Source: three-view drawing plus pictorial views. Frame: mm from the lowest corner of the part. A direction names the side the tool comes from. Give positions to 0.01 mm unless a question says otherwise; leave off trailing zeros. Write each loop counter-clockwise with the first axis right and the second up, starting at its lowest first coordinate (ties: lowest second). Pieces come first, ordered by that corner, then holes. Notation, with made-up numbers: (-20.5, 12.25) -> (24.5, 12.25) arc R22 cw to (24.5, 23.25) -> close; hole circle Ø6 at (2, -32.75). An arc over 180 degrees is marked (long way). Write item = value, one per line.
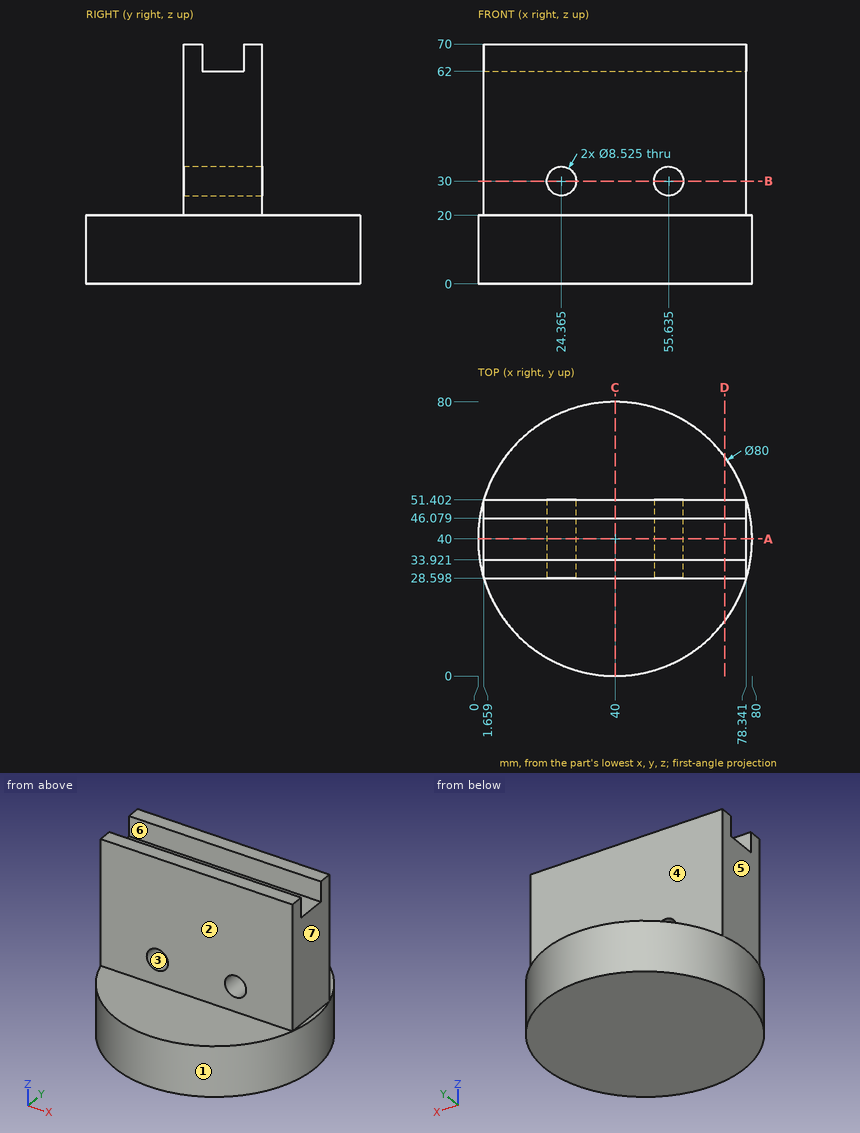
1) Contact query for flat-ended pins moving along their axis: pin 1 (5 mm diameter, centred on x = 11.5, z = 25, fed in from +Y); pin 2 (0.5 mm diameter, centred on x = 1, y = 38.5, fed in from +Z); pin 3 (11.5 mm diameter, centred on y = 36, z = 56, fed in from -X). Output: stop coordinate, or through.
Computed:
pin_1 = 51.4
pin_2 = 20
pin_3 = 1.66
2) Access query for the marked faces 4, 5, 6 and 7. Directions: +Z, -Z, +X, -X, +Y, -Y. A direction counts if a zero-diameter tool reaches every point of the face in a straight line with its end or side. Return the directions, or none.
Computed:
face_4 = +Z, +X, -X, +Y
face_5 = +Z, -X, +Y, -Y
face_6 = +Z, +X, -X
face_7 = +Z, +X, +Y, -Y
3) Cut plane A-A (y = 40). Return the cut outline in (x, z) (1 decimal), then the cut area to 3 significant figures.
Computed:
outline = (0, 0) -> (80, 0) -> (80, 20) -> (78.3, 20) -> (78.3, 62) -> (1.7, 62) -> (1.7, 20) -> (0, 20) -> close; hole circle Ø8.5 at (24.4, 30); hole circle Ø8.5 at (55.6, 30)
area = 4,710 mm²
4) Cut plane D-D (x = 72). Return the cut outline in (y, z).
Computed:
outline = (16, 0) -> (64, 0) -> (64, 20) -> (51.4, 20) -> (51.4, 70) -> (46.08, 70) -> (46.08, 62) -> (33.92, 62) -> (33.92, 70) -> (28.6, 70) -> (28.6, 20) -> (16, 20) -> close
5) Cut plane C-C (x = 40). Return the cut outline in (y, z), then the cut area to 3 significant figures.
Computed:
outline = (0, 0) -> (80, 0) -> (80, 20) -> (51.4, 20) -> (51.4, 70) -> (46.08, 70) -> (46.08, 62) -> (33.92, 62) -> (33.92, 70) -> (28.6, 70) -> (28.6, 20) -> (0, 20) -> close
area = 2,640 mm²
6) Cut plane B-B (z = 30). Return the cut outline in (x, y), then the cut area to 3 significant figures.
Computed:
outline = (1.66, 28.6) -> (20.1, 28.6) -> (20.1, 51.4) -> (1.66, 51.4) -> close; (28.63, 28.6) -> (51.37, 28.6) -> (51.37, 51.4) -> (28.63, 51.4) -> close; (59.9, 28.6) -> (78.34, 28.6) -> (78.34, 51.4) -> (59.9, 51.4) -> close
area = 1,360 mm²
7) Draft query along X for the marked faces 1, 2 and 3. Return one class per face: pulls with the +X half, pulls with the -X half, needs draft (parallel to the pull), parting line crosses it, or undercut.
Computed:
face_1 = parting line crosses it
face_2 = needs draft
face_3 = undercut
8) Material intervals for L1, parallel to Z at x = 27, y = 72.5; L2, parallel to Y at x = 5.5, z = 21; L3, parallel to Z at x = 68.5, y = 40, sorted ascending.
Computed:
L1 = 0 to 20
L2 = 28.6 to 51.4
L3 = 0 to 62
